Source: three-view drawing plus pictorial views. Frame: mm from the lowest corner of the part. Give positions to 0.01 mm unless a question says otherwise; leave off trailing zeros. Loops run counter-clockwise (first coordinate to the right, second up) from the corner with the lowest first, then second, coordinate; pieces in that order, holes last. Notation, with made-up numbers: (38, -5) -> (60, -5) arc R19 ccw to (60, 32) -> close; hole circle Ø5 at (-19, 33.5). An arc over 180 degrees is marked (long way). Answer as a JSON object with one key per item and string values. Group by question number.
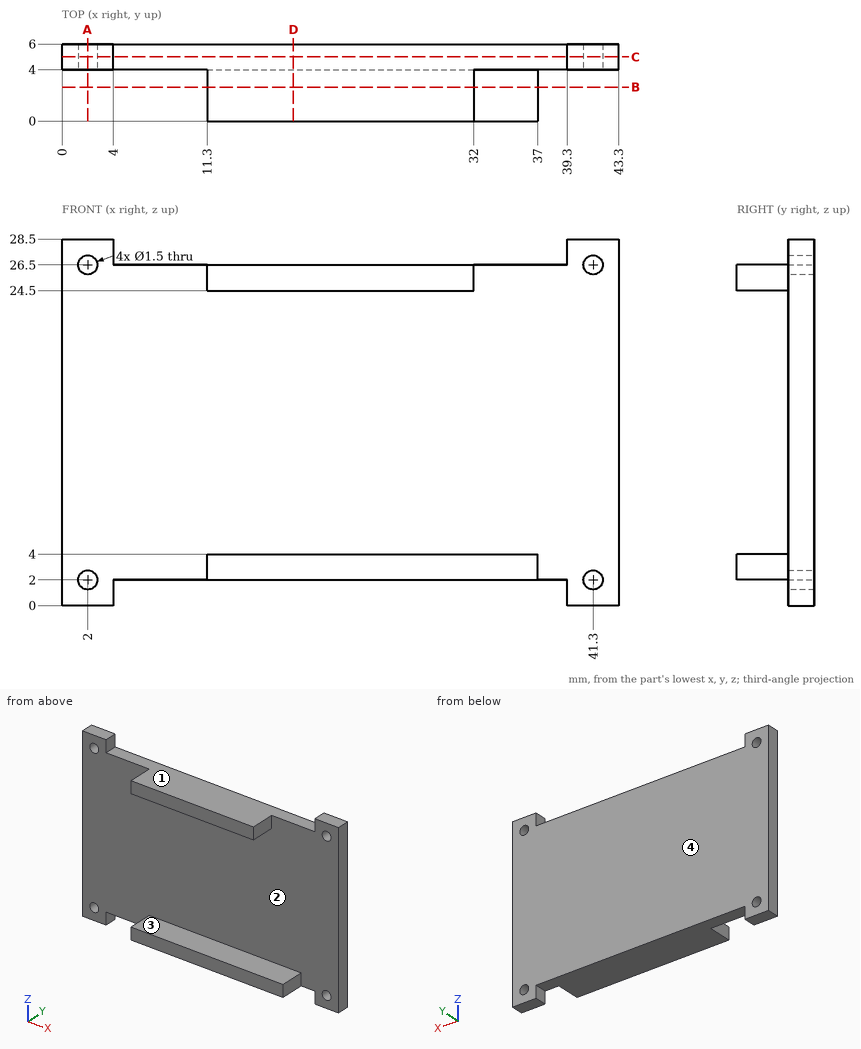
(1) Section query B-B on y = 2.65. Return the cut outline in (x, z), plus the area to 3 significant figures.
(2) Section query D-D on x = 18. Return the cut outline in (y, z).
(3) First-contact query: pin 1 (2 mm diameter, centred on y = 1.5, z = 25.5, fed in from -X); pin 2 (1.2 mm diameter, centred on x = 26, y = 2, fed in from +Z); pin 3 (2 mm diameter, centred on x = 36.5, z = 12.5, fed in from -Y). Flat tips, straight axial feed; report the tip coordinate or a pass-through.
(4) Material intervals for line 1 (Z direction, x = 41.3, y = 4.75); line 2 (Z direction, x = 19.5, y = 1.7); line 3 (Y direction, x = 17, z = 24.25), sorted ascending. Write a range as from..to.
(5) Section query C-C on y = 5. Return the cut outline in (x, z), plus the area to 3 significant figures.
(6) Section query A-A on x = 2. Return the cut outline in (y, z), plus the area to 3 significant figures.
(7) Mould query, pull axis Z, two halves, no side actions, for the marked faces 1, 2, 3 and 4. Classes: pulls with the +Z half, pulls with the -Z half, needs draft (parallel to the pull), parting line crosses it, or undercut.
Result:
{
 "1": {"outline": "(11.3, 2) -> (37, 2) -> (37, 4) -> (11.3, 4) -> close; (11.3, 24.5) -> (32, 24.5) -> (32, 26.5) -> (11.3, 26.5) -> close", "area": "92.8 mm²"},
 "2": {"outline": "(0, 2) -> (6, 2) -> (6, 26.5) -> (0, 26.5) -> (0, 24.5) -> (4, 24.5) -> (4, 4) -> (0, 4) -> close"},
 "3": {"pin 1": "x = 11.3", "pin 2": "z = 26.5", "pin 3": "y = 4"},
 "4": {"line 1": "0..1.25, 2.75..25.75, 27.25..28.5", "line 2": "2..4, 24.5..26.5", "line 3": "4..6"},
 "5": {"outline": "(0, 0) -> (4, 0) -> (4, 2) -> (39.3, 2) -> (39.3, 0) -> (43.3, 0) -> (43.3, 28.5) -> (39.3, 28.5) -> (39.3, 26.5) -> (4, 26.5) -> (4, 28.5) -> (0, 28.5) -> close; hole circle Ø1.5 at (2, 2); hole circle Ø1.5 at (2, 26.5); hole circle Ø1.5 at (41.3, 2); hole circle Ø1.5 at (41.3, 26.5)", "area": "1,090 mm²"},
 "6": {"outline": "(4, 0) -> (6, 0) -> (6, 1.25) -> (4, 1.25) -> close; (4, 2.75) -> (6, 2.75) -> (6, 25.75) -> (4, 25.75) -> close; (4, 27.25) -> (6, 27.25) -> (6, 28.5) -> (4, 28.5) -> close", "area": "51.0 mm²"},
 "7": {"face 1": "pulls with the +Z half", "face 2": "undercut", "face 3": "undercut", "face 4": "needs draft"}
}
